```python
from build123d import *

# Parameters (mm, degrees)
SKETCH1_R           = 2
SKETCH1_R_2         = 7.01
BOSS_EXTRUDE1_DEPTH = 10
CUT_EXTRUDE1_DEPTH  = 10


with BuildPart() as part:
    # Sketch1 → Boss-Extrude1 (new body)
    # profile 1 of 2: a face of its own
    with BuildSketch(Plane(origin=(0, 0, 0), x_dir=(1, 0, 0), z_dir=(0, 1, 0))):
        with BuildLine():
            ThreePointArc((0, 16.5), (-16.5, 0), (0, -16.5))
            ThreePointArc((0, -16.5), (11.66726189, -11.66726189), (16.5, 0))
            ThreePointArc((16.5, 0), (14.076910684, 8.607588837), (7.519322958, 14.68706173))
            Line((7.519322958, 14.68706173), (0, 16.5))
        make_face()
        with Locations(Location((0, -11.314, 0), (0, 0, 270))):
            Circle(SKETCH1_R, mode=Mode.SUBTRACT)
        with Locations(Location((-11.314, 0, 0), (0, 0, 270))):
            Circle(SKETCH1_R, mode=Mode.SUBTRACT)
        with Locations(Location((0, 0, 0), (0, 0, 270))):
            Circle(SKETCH1_R_2, mode=Mode.SUBTRACT)
        with Locations(Location((11.314, 0, 0), (0, 0, 270))):
            Circle(SKETCH1_R, mode=Mode.SUBTRACT)
        with Locations(Location((0, 11.314, 0), (0, 0, 270))):
            Circle(SKETCH1_R, mode=Mode.SUBTRACT)
    # profile 2 of 2: a face of its own
    with BuildSketch(Plane(origin=(0, 0, 0), x_dir=(1, 0, 0), z_dir=(0, 1, 0))):
        with BuildLine():
            ThreePointArc((16.5, 0), (11.66726189, -11.66726189), (0, -16.5))
            Line((0, -16.5), (19.087841457, -16.5))
            Line((19.087841457, -16.5), (42.57033822, -16.5))
            Line((42.57033822, -16.5), (65.434874542, -16.5))
            Line((65.434874542, -16.5), (65.529162168, -16.5))
            Line((65.529162168, -16.5), (70, -29.789637879))
            Line((70, -29.789637879), (81.21126045, -29.789637879))
            Line((81.21126045, -29.789637879), (80.86351064, -16.5))
            Line((80.86351064, -16.5), (80.641091233, -8))
            Line((80.641091233, -8), (80.507921559, -2.910775794))
            Line((80.507921559, -2.910775794), (7.519322958, 14.68706173))
            ThreePointArc((7.519322958, 14.68706173), (14.076910684, 8.607588837), (16.5, 0))
        make_face()
    extrude(amount=BOSS_EXTRUDE1_DEPTH)

    # Sketch2 → Cut-Extrude1 (cut)
    with BuildSketch(Plane(origin=(0, 10, 0), x_dir=(1, 0, 0), z_dir=(0, 1, 0))):
        with BuildLine():
            add(Edge.make_bspline(
                [(0, -16.5), (14.394754893, -15.656765563), (16.5, 0)],
                knots=[0, 0, 0, 1, 1, 1], degree=2))
            Line((0, -16.5), (43.395579658, -16.5))
            Line((43.395579658, -16.5), (43.395579658, -11.239382549))
            Line((43.395579658, -11.239382549), (38.779311098, -3.023634866))
            Line((38.779311098, -3.023634866), (16.5, 2.347994462))
            Line((16.5, 2.347994462), (16.5, 0))
        make_face()
        Polygon((42.670487587, 0.800617581), (49.435529091, -11.239382549), (72.209122235, -11.239382549), (71.607948341, -6.176317755), align=None)
    extrude(amount=-CUT_EXTRUDE1_DEPTH, mode=Mode.SUBTRACT)


solid = part.part
```
Here's how the part is built. I have some questions about the finished solid (model axes, mm). A direction names the side the tool comes from. Coordinates: 2 decimals unless noted, no trailing zeros. Loops run counter-clockwise (first coordinate to the right, second up) from the corner with the lowest first, then second, coordinate; pieces in that order, holes last. Notation, with made-up numbers: (14, -12.75) - (45, -12.75) arc R25 ccw to (45, 15.25) - close; hole circle Ø7 at (80.25, 18). An arc over 180 degrees is marked (long way). Return JSON: item names as keys, results as strings. Group by question number.
Item 1: On a 3-axis mill with a long thin cutter (end or side, diameter ignored), from which of +Z, -Z, +X, -X, +Y, -Y can I reach the whole of each face in a straight line? I mean faces 5 (the face through (54, 5, 16.5)), 6 (the face through (27.796, 5.07, 0.375)), 7 (the face through (76, 5, 29.79)), 8 (the face through (57.342, 5.07, 2.737)), 9 (the face through (32, 10, 0)). Say none if no direction works.
Item 2: If we section it at B-B on z = 23: Write out the boundary of the cut face in (x, y), and give its area (3 significant figures).
Item 3: We'd pull the mould along Z, two halves only. Please class faces 1 (the face through (-1.22, 4.93, -12.9)), 2 (the face through (43.396, 5, 14)), 3 (the face through (41.12, 5.07, 7.19)), 4 (the face through (-9.33, 4.93, -0.26)): +Z half, -Z half, draft (parallel to the pull), parting line (faces both ways), or undercut.
Item 4: If we section it at C-C on z = 1: State how many separate pieces and enclosed holes the cut face has, and give its area (3 significant figures).
Item 5: I need wall thicknesses on line 1 (X direction, y = 3.5, z = 12); line 2 (Z direction, x = -4, y = 5.75); line 3 (X direction, y = 4.25, z = 9). Which ranges of each line are inside material? Lowest first, please. Write a range as from..to.
Item 6: Will these pins go through, and if not, where does the flat tip stop? P1, Ø2.5, axis at x = 11.314, z = 0, coming from the +Y side; P2, Ø5, axis at x = 54.5, y = 3, coming from the +Z side; P3, Ø2.5, axis at y = 3, z = 13.5, coming from the -X side; P4, Ø2, axis at x = 56, y = 4, coming from the -Z side.
Item 7: If we section it at A-A on x = 58: Write out the boundary of the cut face in (y, z).
Calculated:
{
 "1": {"face 5": "+Z, -X, +Y, -Y", "face 6": "+Z, +Y, -Y", "face 7": "+Z, +X, -X, +Y, -Y", "face 8": "+Y, -Y", "face 9": "+Z, -Z, +X, -X, +Y"},
 "2": {"outline": "(67.72, 0) - (81.03, 0) - (81.03, 10) - (67.72, 10) - close", "area": "133 mm^2"},
 "3": {"face 1": "undercut", "face 2": "draft", "face 3": "+Z half", "face 4": "undercut"},
 "4": {"separate pieces": "6", "enclosed holes": "0", "area": "478 mm^2"},
 "5": {"line 1": "x = -11.32..-1.88, 1.88..11.28, 43.4..80.75", "line 2": "z = -16.01..-5.76, 5.76..16.01", "line 3": "x = -13.83..13.61, 42.14..48.18, 71.94..80.67"},
 "6": {"P1": "passes through", "P2": "stops at z = 16.5", "P3": "stops at x = -11.05", "P4": "stops at z = -3.24"},
 "7": {"outline": "(0, -2.52) - (10, -2.52) - (10, 2.9) - (0, 2.9) - close; (0, 11.24) - (10, 11.24) - (10, 16.5) - (0, 16.5) - close"}
}
